Study the drawing (mm; zero at the part's minimum x, y, z) and answer. A direction names the side the tool comes from. Give positions to 0.01 mm unless a question says otherwise; leave off trailing zeros. Loops run counter-clockwise (first coordinate to the right, second up) from the corner with the lowest first, then second, coordinate; pieces in that order, holes last. Notation, with made-up numbers: (24.5, 25.5) - (56.5, 25.5) arc R5 cw to (56.5, 32.5) - close; hole circle Ø9 at (-10.5, -10). An arc over 180 degrees is marked (long way). Use one line per item in the form item = value. Start each with the question number.
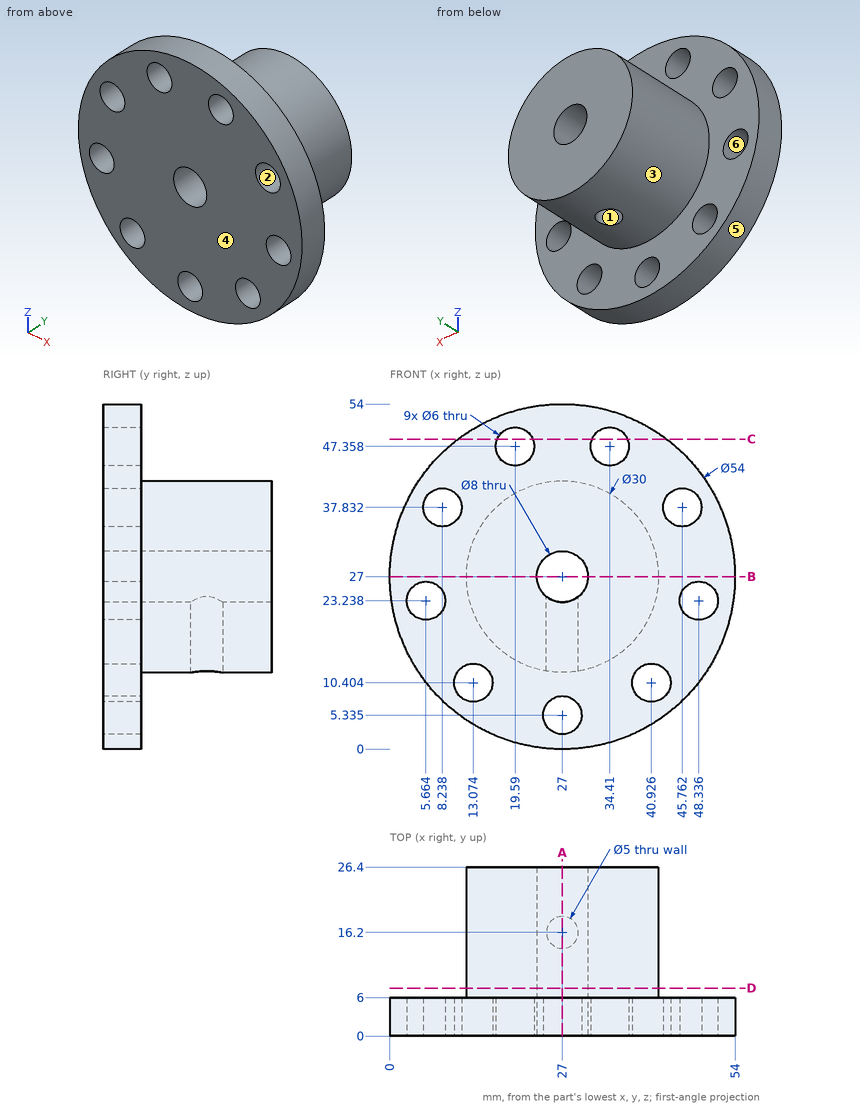
1) A tool of negligible diameter and unlimited length cuts with its end or side. For the marked faces 1, 2 and 3, from which of +Z, -Z, +X, -X, +Y, -Y can it reach the whole face along a straight path? Write none if from no direction.
2) Find the intervals of material crossed by probe 1 along X at (y, z) = (15, 27); probe 2 along Y at (x, z) = (23.5, 49.5); probe 3 along X at (y, z) = (25, 25) (1 decimal), in increasing order.
3) Flat-ended cylindrical pins translate along their axes: pin 1 Ø8 at (x, z) = (40.93, 10.4) entering from +Y; pin 2 Ø8 at (x, z) = (34.41, 47.36) entering from -Y; pin 3 Ø3 at (x, y) = (27, 16.2) entering from +Z; pin 4 Ø4 at (x, y) = (23, 9) entering from -Z. Find the tip coordinate at first contact, or state that the pin passes through.
4) A cutting plane is placed at A-A (x = 27). Give the vertices of the cut face in (y, z) (1 decimal), plus the area to 3 significant figures.
5) Determine the mould class of the marked faces 4, 5 and 6 for opening direction X: released by +X, released by -X, zero draft, split by the parting line, or undercut.
6) A cutting plane is placed at C-C (z = 48.5). Give the vertices of the cut face in (x, y) (1 decimal).
7) A cutting plane is placed at B-B (z = 27). Give the vertices of the cut face in (x, y), plus the area to 3 significant figures.
8) A cutting plane is placed at D-D (y = 7.5). Give the vertices of the cut face in (x, z).
Answer sheet:
q1.face_1 = -Z
q1.face_2 = +Y, -Y
q1.face_3 = +Y
q2.probe_1 = 12 to 23, 31 to 42
q2.probe_2 = 0 to 6
q2.probe_3 = 12.1 to 23.5, 30.5 to 41.9
q3.pin_1 = 6
q3.pin_2 = 0
q3.pin_3 = 42
q3.pin_4 = 12.13
q4.outline = (0, 0) - (6, 0) - (6, 2.3) - (0, 2.3) - close; (0, 8.3) - (6, 8.3) - (6, 12) - (13.7, 12) - (13.7, 23) - (0, 23) - close; (0, 31) - (26.4, 31) - (26.4, 42) - (6, 42) - (6, 54) - (0, 54) - close; (18.7, 12) - (26.4, 12) - (26.4, 23) - (18.7, 23) - close
q4.area = 634 mm²
q5.face_4 = zero draft
q5.face_5 = split by the parting line
q5.face_6 = undercut
q6.outline = (10.7, 0) - (16.8, 0) - (16.8, 6) - (10.7, 6) - close; (22.4, 0) - (31.6, 0) - (31.6, 6) - (22.4, 6) - close; (37.2, 0) - (43.3, 0) - (43.3, 6) - (37.2, 6) - close
q7.outline = (0, 0) - (23, 0) - (23, 26.4) - (12, 26.4) - (12, 6) - (0, 6) - close; (31, 0) - (54, 0) - (54, 6) - (42, 6) - (42, 26.4) - (31, 26.4) - close
q7.area = 725 mm²
q8.outline = circle Ø30 at (27, 27); hole circle Ø8 at (27, 27)
